```python
from build123d import *

# Parameters (mm, degrees)
SKETCH1_R               = 7.5
BOSS_EXTRUDE1_DEPTH     = 58
SKETCH2_W               = 38
SKETCH2_H               = 30
CUT_EXTRUDE1_DEPTH      = 84.865217872
CUT_EXTRUDE1_DEPTH_BACK = 84.865217872
SKETCH3_W               = 16
SKETCH3_H               = 6
CUT_EXTRUDE4_DEPTH      = 84.865217872
CUT_EXTRUDE4_DEPTH_BACK = 84.865217872
SKETCH4_R               = 7
CUT_EXTRUDE5_DEPTH      = 100.435906681
CUT_EXTRUDE5_DEPTH_BACK = 100.435906681
CUT_EXTRUDE6_DEPTH      = 84.865217872
CUT_EXTRUDE6_DEPTH_BACK = 84.865217872


with BuildPart() as part:
    # Sketch1 → Boss-Extrude1 (new body)
    with BuildSketch(Plane.XY):
        with BuildLine():
            Line((32.5, -19), (-32.5, -19))
            Line((-32.5, -19), (-32.5, 5))
            ThreePointArc((-32.5, 5), (-15.83939444, 16.82575695), (4.16060556, 21))
            Line((4.16060556, 21), (32.5, 21))
            Line((32.5, 21), (45.490381057, 13.5))
            Line((45.490381057, 13.5), (45.490381057, -11.5))
            Line((45.490381057, -11.5), (32.5, -19))
        make_face()
        with Locations(Location((0, 0, 0), (0, 0, 180))):
            Circle(SKETCH1_R, mode=Mode.SUBTRACT)
    extrude(amount=BOSS_EXTRUDE1_DEPTH)

    # Sketch2 → Cut-Extrude1 (cut, two sides)
    with BuildSketch(Plane(origin=(0, 21, 0), x_dir=(1, 0, 0), z_dir=(0, 1, 0))) as cut_extrude1_sk:
        with Locations((2.5, -29)):
            Rectangle(SKETCH2_W, SKETCH2_H)
    extrude(amount=CUT_EXTRUDE1_DEPTH, mode=Mode.SUBTRACT)
    extrude(cut_extrude1_sk.sketch, amount=-CUT_EXTRUDE1_DEPTH_BACK, mode=Mode.SUBTRACT)

    # Sketch3 → Cut-Extrude4 (cut, two sides)
    with BuildSketch(Plane(origin=(0, 21, 0), x_dir=(1, 0, 0), z_dir=(0, 1, 0))) as cut_extrude4_sk:
        with Locations((-24.5, -47)):
            Rectangle(SKETCH3_W, SKETCH3_H)
        with Locations((-24.5, -11)):
            Rectangle(SKETCH3_W, SKETCH3_H)
    extrude(amount=CUT_EXTRUDE4_DEPTH, mode=Mode.SUBTRACT)
    extrude(cut_extrude4_sk.sketch, amount=-CUT_EXTRUDE4_DEPTH_BACK, mode=Mode.SUBTRACT)


with BuildPart() as body_2:
    # of the pieces the cut leaves, the one that is kept (cut_extrude4_keep)
    add(part.part.solids().sort_by_distance((4.16060556, 21, 0))[0])

    # Sketch4 → Cut-Extrude5 (cut, two sides)
    with BuildSketch(Plane(origin=(45.490381057, 0, 0), x_dir=(0, 0, -1), z_dir=(1, 0, 0))) as cut_extrude5_sk:
        with Locations(Location((-29, 0, 0), (0, 0, 90))):
            Circle(SKETCH4_R)
    extrude(amount=CUT_EXTRUDE5_DEPTH, mode=Mode.SUBTRACT)
    extrude(cut_extrude5_sk.sketch, amount=-CUT_EXTRUDE5_DEPTH_BACK, mode=Mode.SUBTRACT)

    # Sketch6 → Cut-Extrude6 (cut, two sides)
    with BuildSketch(Plane(origin=(0, 21, 0), x_dir=(1, 0, 0), z_dir=(0, 1, 0))) as cut_extrude6_sk:
        Polygon((32.5, 0), (45.490381057, -12.990381057), (45.490381057, 0), align=None)
        Polygon((45.490381057, -45.009618943), (45.490381057, -58), (32.5, -58), align=None)
    extrude(amount=CUT_EXTRUDE6_DEPTH, mode=Mode.SUBTRACT)
    extrude(cut_extrude6_sk.sketch, amount=-CUT_EXTRUDE6_DEPTH_BACK, mode=Mode.SUBTRACT)


solid = body_2.part
```
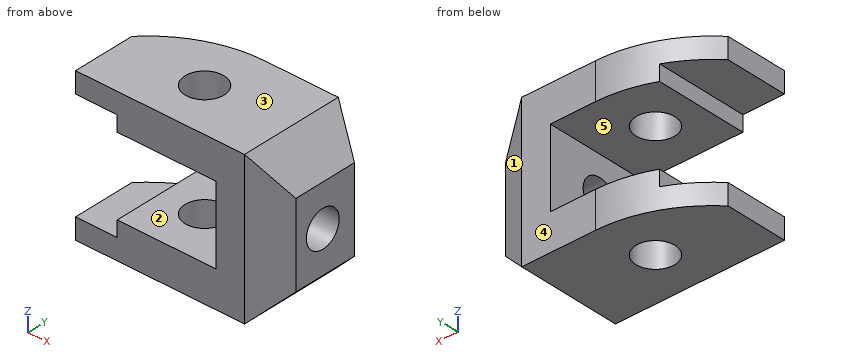
Verification items for the finished model (mm, model axes). Face numbers are marked on the shaded views. A direction names the side the tool comes from. Give positions to 0.01 mm unless a question says otherwise; leave off trailing zeros. Write each loop counter-clockwise with the first axis right and the second up, starting at its lowest first coordinate (ties: lowest second). Pieces come first, ordered by that corner, then holes. Notation, with made-up numbers: (66, 85.25) - (107, 85.25) arc R27 ccw to (107, 108.25) - close; hole circle Ø6 at (-6.75, 3). An arc over 180 degrees is marked (long way). Put each result on its own line as item: value.
Q1. Section check A-A on y = 0. Record the cut outline in (x, z).
Result:
outline: (-32.5, 0) - (-7.5, 0) - (-7.5, 14) - (-16.5, 14) - (-16.5, 8) - (-32.5, 8) - close; (-32.5, 50) - (-16.5, 50) - (-16.5, 44) - (-7.5, 44) - (-7.5, 58) - (-32.5, 58) - close; (7.5, 0) - (32.5, 0) - (45.49, 12.99) - (45.49, 22) - (21.5, 22) - (21.5, 14) - (7.5, 14) - close; (7.5, 44) - (21.5, 44) - (21.5, 36) - (45.49, 36) - (45.49, 45.01) - (32.5, 58) - (7.5, 58) - close
Q2. Mould release check, pull along Z, two halves, no side actions. Record for the marked faces 3, 4 and 5: released by +Z, released by -Z, zero draft, split by the parting line, or undercut.
Result:
face 3: released by +Z
face 4: zero draft
face 5: undercut
Q3. Section check C-C on x = -2. Record the cut outline in (y, z).
Result:
outline: (-19, 0) - (-7.23, 0) - (-7.23, 14) - (-19, 14) - close; (-19, 44) - (-7.23, 44) - (-7.23, 58) - (-19, 58) - close; (7.23, 0) - (20.62, 0) - (20.62, 14) - (7.23, 14) - close; (7.23, 44) - (20.62, 44) - (20.62, 58) - (7.23, 58) - close
Q4. Section check D-D on z = 10.5. Record the cut outline in (x, y).
Result:
outline: (-16.5, -19) - (32.5, -19) - (43, -12.94) - (43, 14.94) - (32.5, 21) - (4.16, 21) arc R50 ccw to (-16.5, 16.53) - close; hole circle Ø15 at (0, 0)
Q5. Section check B-B on z = 29. Record the cut outline in (x, y), and give its area (3 significant figures).
Result:
outline: (21.5, -19) - (32.5, -19) - (45.49, -11.5) - (45.49, -7) - (21.5, -7) - close; (21.5, 7) - (45.49, 7) - (45.49, 13.5) - (32.5, 21) - (21.5, 21) - close
area: 526 mm2
Q6. Scan lines: probe 1 along Z at (x, y) = (30.5, 0); probe 2 along Z at (x, y) = (2.5, -7.5); probe 3 along X at (y, z) = (-5, 15.5). Record each from-to range of solid material in increasing order. Write a range as from..to.
Result:
probe 1: 0..22, 36..58
probe 2: 0..14, 44..58
probe 3: 21.5..45.49
Q7. Depth check by flat-ended pin: P1, Ø1.8, axis at y = 5, z = 11, coming from the -X side; P2, Ø8.5, axis at y = 0, z = 29, coming from the +X side; P3, Ø5, axis at x = 35.5, z = 43, coming from the +Y side; P4, Ø1, axis at x = -3, z = 52, coming from the +Y side. Enter the tip coordinate at first touch or a pass-through.
Result:
P1: x = -16.5
P2: through
P3: y = 20.71
P4: y = 20.55
Q8. Set-up check for the marked faces 1 and 2: record each of +Z, -Z, +X, -X, +Y, -Y from which the full face is reachable in a straight line by a thin tool's end or side.
Result:
face 1: +Z, -Z, +X, +Y
face 2: -X, +Y, -Y
